from build123d import *

# Parameters (mm, degrees)
F0_R      = 11.050187
F1_DEPTH  = 152.4
F2_R      = 10.16
F3_R      = 1.293734
F4_DEPTH  = 76.2
F5_R      = 8.49004
F5_R_2    = 1.449468
F6_DEPTH  = 15.24
F7_R      = 7.435283
F7_R_2    = 1.669858
F8_DEPTH  = 12.7
F9_R      = 21.64415
F10_DEPTH = 1.524


with BuildPart() as f1:
    # F0 (on Top) → F1 (new body)
    with BuildSketch(Plane.XY):
        Circle(F0_R)
    extrude(amount=F1_DEPTH)

    # F2
    f2_edges = [f1.edges().sort_by_distance(p)[0] for p in [
        (-11.050187, 0, 152.4),
    ]]
    fillet(f2_edges, radius=F2_R)

    # F3 (on face) → F4 (join)
    with BuildSketch(Plane(origin=(0, 0, 0), x_dir=(1, 0, 0), z_dir=(0, 0, -1))):
        Circle(F3_R)
    extrude(amount=F4_DEPTH)

    # F5 (on face) → F6 (join)
    with BuildSketch(Plane(origin=(0, 0, 0), x_dir=(1, 0, 0), z_dir=(0, 0, -1))):
        Circle(F5_R)
        Circle(F5_R_2, mode=Mode.SUBTRACT)
    extrude(amount=F6_DEPTH)

    # F7 (on face) → F8 (cut)
    with BuildSketch(Plane(origin=(0, 0, -15.24), x_dir=(1, 0, 0), z_dir=(0, 0, -1))):
        Circle(F7_R)
        Circle(F7_R_2, mode=Mode.SUBTRACT)
    extrude(amount=-F8_DEPTH, mode=Mode.SUBTRACT)

    # F9 (on face) → F10 (join)
    with BuildSketch(Plane(origin=(0, 0, -76.2), x_dir=(1, 0, 0), z_dir=(0, 0, -1))):
        Circle(F9_R)
    extrude(amount=F10_DEPTH)


solid = f1.part
Check sheet for the modelled part. Datum: model origin and axes. Units: mm. A direction names the side the tool comes from. Give positions to 0.01 mm unless a question says otherwise; leave off trailing zeros. Write each loop counter-clockwise with the first axis right and the second up, starting at its lowest first coordinate (ties: lowest second). Pieces come first, ordered by that corner, then holes. Notation, with made-up numbers: (61, -4) -> (117, -4) arc R18 cw to (117, 13) -> close; hole circle Ø6 at (74.25, 3.25). An arc over 180 degrees is marked (long way). Use one line per item in the form item = value. Start each with the question number.
1. Section check A-A (z = -6.5). Record the cut outline in (x, y), and give its area (3 significant figures).
2. Thickness scan on line 1 along Y through (x, z) = (0, -7); line 2 along Z through (x, y) = (-2.5, 9). Record the ranges inside material, lowest first. Write a range as from..to.
3. Access from +Z, -Z, +X, -X, +Y, -Y to the whole of each face (thin tool, end or side, straight path). Record for faces 1 (the flat face through (0, 0, -77.724)), 2 (the cylindrical face through (-2.395, -10.787, 70.124)), 3 (the flat face through (3.2, -8.1, 0)).
4. Section check C-C (y = 17.5). Record the cut outline in (x, z).
5. Mould release check, pull along Y, two halves, no side actions. Record for faces 4 (the flat face through (0, 8, -15.24)), 5 (the flat face through (0, -2, -2.54)), 6 (the cylindrical face through (-1.61, 7.26, -8.98)), 7 (the cylindrical face through (-4.69, 21.13, -76.95)): pulls with the +Y half, pulls with the -Y half, needs draft (parallel to the pull), parting line crosses it, or undercut.
6. Section check D-D (z = 32). Record the cut outline in (x, y), and give its area (3 significant figures).
7. Go/stop test with flat-tipped pins: P1, Ø12, axis at x = 11.5, z = -7, coming from the +Y side; P2, Ø1, axis at y = -1.5, z = 23, coming from the +X side; P3, Ø10, axis at x = 10, y = 16.5, coming from the +Z side. Record where each tip stops, or that it passes through.
8. Section check B-B (x = -18). Record the cut outline in (y, z).
Conclusion:
q1.outline = circle Ø16.98 at (0, 0); circle Ø3.34 at (0, 0); circle Ø2.59 at (0, 0); hole circle Ø14.87 at (0, 0); hole circle Ø2.9 at (0, 0)
q1.area = 60.2 mm²
q2.line_1 = -8.49..-7.44, -1.67..-1.45, -1.29..1.29, 1.45..1.67, 7.44..8.49
q2.line_2 = -77.72..-76.2, 0..147.88
q3.face_1 = -Z, +X, -X, +Y, -Y
q3.face_2 = +Z
q3.face_3 = none
q4.outline = (-12.74, -77.72) -> (12.74, -77.72) -> (12.74, -76.2) -> (-12.74, -76.2) -> close
q5.face_4 = needs draft
q5.face_5 = undercut
q5.face_6 = undercut
q5.face_7 = parting line crosses it
q6.outline = circle Ø22.1 at (0, 0)
q6.area = 384 mm²
q7.P1 = 6.47
q7.P2 = 11
q7.P3 = -76.2
q8.outline = (-12.02, -77.72) -> (12.02, -77.72) -> (12.02, -76.2) -> (-12.02, -76.2) -> close
